Check sheet for the modelled part. Datum: model origin and axes. Units: mm. A direction names the side the tool comes from. Give positions to 0.01 mm unless a question says otherwise; leave off trailing zeros. Order: outer loops, then holes, each group sorted by start corner. A loop starts at its lowest first (then second) coordinate and runs counter-clockwise, first axis right, second up.
```python
from build123d import *

# Parameters (mm, degrees)
F0_R     = 25
F0_R_2   = 20
F0_R_3   = 13.5
F0_R_4   = 10
F0_R_5   = 7
F1_DEPTH = 5
F2_DEPTH = 40
F3_DEPTH = 40


with BuildPart() as f1:
    # F0 (on Top) → F1 (new body)
    with BuildSketch(Plane.XY):
        Circle(F0_R)
        Circle(F0_R_2, mode=Mode.SUBTRACT)
        Circle(F0_R_2)
        Circle(F0_R_3, mode=Mode.SUBTRACT)
        Circle(F0_R_3)
        Circle(F0_R_4, mode=Mode.SUBTRACT)
        Circle(F0_R_4)
        Circle(F0_R_5, mode=Mode.SUBTRACT)
    extrude(amount=F1_DEPTH)

    # F0 (on Top) → F2 (join)
    with BuildSketch(Plane.XY):
        Circle(F0_R_2)
        Circle(F0_R_3, mode=Mode.SUBTRACT)
    extrude(amount=F2_DEPTH)

    # F0 (on Top) → F3 (join)
    with BuildSketch(Plane.XY):
        Circle(F0_R_4)
        Circle(F0_R_5, mode=Mode.SUBTRACT)
    extrude(amount=F3_DEPTH)


solid = f1.part
```
(1) Gauge pin test, flat ends, axial feed: pin 1 Ø1.5 at (y, z) = (10.5, 30) entering from -X; pin 2 Ø5 at (y, z) = (-11, 21.5) entering from +X; pin 3 Ø4 at (y, z) = (12, 7.5) entering from +X. Record the tip position at first contact, or that the pin passes through.
Response values:
pin 1: stops at x = -17.46
pin 2: stops at x = 18.1
pin 3: stops at x = 17.32
(2) Cross-section at D-D on y = 11. Enter the section's corners in (x, z), then the cut area to 3 significant figures.
Response values:
outline: (-22.45, 0) - (22.45, 0) - (22.45, 5) - (16.7, 5) - (16.7, 40) - (7.83, 40) - (7.83, 5) - (-7.83, 5) - (-7.83, 40) - (-16.7, 40) - (-16.7, 5) - (-22.45, 5) - close
area: 846 mm2
(3) Cross-section at C-C on z = 8. Enter the section's corners in (x, y), then the cut area to 3 significant figures.
Response values:
outline: circle Ø40 at (0, 0); circle Ø20 at (0, 0); hole circle Ø27 at (0, 0); hole circle Ø14 at (0, 0)
area: 844 mm2
(4) Set-up check for faces 1 (the face through (-9, -5, 5)), 2 (the face through (-7, -2, 40)): record each of +Z, -Z, +X, -X, +Y, -Y from which the full face is reachable in a straight line by a thin tool's end or side.
Response values:
face 1: +Z
face 2: +Z, +X, -X, +Y, -Y
(5) Release check for a two-part mould opening along X. For faces 3 (the face through (-2.93, -13.18, 22.26)), 4 (the face through (-4.336, -19.524, 22.255)), 5 (the face through (-2.17, -9.76, 22.26)), 6 (the face through (5.2, -5.2, 0)) record: released by +X, released by -X, zero draft, split by the parting line, or undercut.
Response values:
face 3: undercut
face 4: split by the parting line
face 5: undercut
face 6: zero draft
(6) Cross-section at A-A on y = 0. Enter the section's corners in (x, z).
Response values:
outline: (-25, 0) - (-7, 0) - (-7, 40) - (-10, 40) - (-10, 5) - (-13.5, 5) - (-13.5, 40) - (-20, 40) - (-20, 5) - (-25, 5) - close; (7, 0) - (25, 0) - (25, 5) - (20, 5) - (20, 40) - (13.5, 40) - (13.5, 5) - (10, 5) - (10, 40) - (7, 40) - close
(7) Material ranges on L1, parallel to Y at x = 0, z = 14; L2, parallel to Y at x = -8.5, z = 14; L3, parallel to Z at x = -14, y = 20, recorded low to high.
Response values:
L1: y = -20 to -13.5, -10 to -7, 7 to 10, 13.5 to 20
L2: y = -18.1 to -10.49, -5.27 to 5.27, 10.49 to 18.1
L3: z = 0 to 5
